Could you check a few things on this model? Use its own coordinates, in mm. Coordinates: 2 decimals unless noted, no trailing zeros. Order: outer loops, then holes, each group sorted by start corner. A loop starts at its lowest first (then second) coordinate and runs counter-clockwise, first axis right, second up. Notation, with made-up numbers: (-14.75, -37.75) - (10.25, -37.75) arc R26 cw to (10.25, -18.75) - close; hole circle Ø2 at (6, 48). An arc over 180 degrees is marked (long way). Answer as CSV lines item,"result". Start each with the question number.
1. I want a section at A-A, the plane x = 6.5. List the corners of the cut face in (y, z) for me, and give its area (3 significant figures).
2. For pin 1 (3 mm diameter, centred on x = -46.5, z = -42, fed in from -Y); pin 2 (1.5 mm diameter, centred on y = 8.5, z = -21, fed in from -X); pin 3 (6 mm diameter, centred on x = 30.5, y = 11.5, fed in from +Z); pin 4 (10 mm diameter, centred on x = -22, y = 11.5, fed in from -Z), each with a flat end and sliding along its axis, tell me the tip position at first contact or that it passes through.
3. I want a section at B-B, the plane x = -24.5. List the corners of the cut face in (y, z) for me.
4. I need wall thicknesses on probe 1 along Z at (x, y) = (-27.5, 21.25); probe 2 along X at (y, z) = (9.75, -13.5); probe 3 along X at (y, z) = (4.5, 47). Which ranges of each line are inside material? Lowest first, please.
from build123d import *

# Parameters (mm, degrees)
SKETCH1_R           = 62.5
BOSS_EXTRUDE1_DEPTH = 25
CAVITY1_DEPTH       = 25


# Read off the part's stored shape, not the designer's step: Cavity1
with BuildPart() as part:
    # Sketch1 → Boss-Extrude1 (new body)
    with BuildSketch(Plane(origin=(0, 0, 0), x_dir=(1, 0, 0), z_dir=(0, 1, 0))):
        with Locations(Location((0, 0, 0), (0, 0, 270))):
            Circle(SKETCH1_R)
    extrude(amount=BOSS_EXTRUDE1_DEPTH)

    # Cavity1 outline → Cavity1 (cut)
    with BuildSketch(Plane(origin=(0, 0, 0), x_dir=(1, 0, 0), z_dir=(0, 1, 0))):
        with BuildLine():
            Line((16.350867892, -49.873660473), (20.022970331, -51.745036944))
            ThreePointArc((20.022970331, -51.745036944), (24.456878574, -49.800038203), (28.704396647, -47.476000203))
            Line((28.704396647, -47.476000203), (29.464309883, -43.425207924))
            ThreePointArc((29.464309883, -43.425207924), (30.217762384, -42.903777412), (30.961999914, -42.369276757))
            Line((30.961999914, -42.369276757), (35.032663999, -43.014319485))
            ThreePointArc((35.032663999, -43.014319485), (38.648523661, -39.79436276), (41.969986165, -36.271516008))
            Line((41.969986165, -36.271516008), (41.440942946, -32.18415751))
            ThreePointArc((41.440942946, -32.18415751), (41.996387967, -31.455417996), (42.539030133, -30.717095621))
            Line((42.539030133, -30.717095621), (46.609790903, -30.07266333))
            ThreePointArc((46.609790903, -30.07266333), (49.053656447, -25.89294042), (51.12393549, -21.5161257))
            Line((51.12393549, -21.5161257), (49.357722251, -17.792300112))
            ThreePointArc((49.357722251, -17.792300112), (49.660788964, -16.927585698), (49.94871817, -16.05771374))
            Line((49.94871817, -16.05771374), (53.621101197, -14.186887953))
            ThreePointArc((53.621101197, -14.186887953), (54.653750036, -9.456539258), (55.270192281, -4.654189691))
            Line((55.270192281, -4.654189691), (52.43969828, -1.658411006))
            ThreePointArc((52.43969828, -1.658411006), (52.460720403, -0.742365963), (52.465752134, 0.173906448))
            Line((52.465752134, 0.173906448), (55.380278979, 3.087996269))
            ThreePointArc((55.380278979, 3.087996269), (54.900628251, 7.905931261), (54.002892036, 12.66372824))
            Line((54.002892036, 12.66372824), (50.385185747, 14.63821233))
            ThreePointArc((50.385185747, 14.63821233), (50.122105488, 15.515919131), (49.843747202, 16.388900869))
            Line((49.843747202, 16.388900869), (51.715123672, 20.061003308))
            ThreePointArc((51.715123672, 20.061003308), (49.770124931, 24.49491155), (47.446086932, 28.742429624))
            Line((47.446086932, 28.742429624), (43.395294653, 29.50234286))
            ThreePointArc((43.395294653, 29.50234286), (42.87386414, 30.255795361), (42.339363485, 31.000032891))
            Line((42.339363485, 31.000032891), (42.984406214, 35.070696976))
            ThreePointArc((42.984406214, 35.070696976), (39.764449489, 38.686556638), (36.241602736, 42.008019142))
            Line((36.241602736, 42.008019142), (32.154244239, 41.478975923))
            ThreePointArc((32.154244239, 41.478975923), (31.425504725, 42.034420944), (30.68718235, 42.57706311))
            Line((30.68718235, 42.57706311), (30.042750059, 46.64782388))
            ThreePointArc((30.042750059, 46.64782388), (25.863027148, 49.091689424), (21.486212429, 51.161968467))
            Line((21.486212429, 51.161968467), (17.762386841, 49.395755228))
            ThreePointArc((17.762386841, 49.395755228), (16.897672427, 49.698821941), (16.027800469, 49.986751147))
            Line((16.027800469, 49.986751147), (14.156974682, 53.659134174))
            ThreePointArc((14.156974682, 53.659134174), (9.426625987, 54.691783013), (4.62427642, 55.308225258))
            Line((4.62427642, 55.308225258), (1.628497735, 52.477731257))
            ThreePointArc((1.628497735, 52.477731257), (0.712452692, 52.49875338), (-0.20381972, 52.503785111))
            Line((-0.20381972, 52.503785111), (-3.11790954, 55.418311956))
            ThreePointArc((-3.11790954, 55.418311956), (-7.935844532, 54.938661228), (-12.693641511, 54.040925013))
            Line((-12.693641511, 54.040925013), (-14.668125602, 50.423218724))
            ThreePointArc((-14.668125602, 50.423218724), (-15.545832402, 50.160138465), (-16.41881414, 49.881780179))
            Line((-16.41881414, 49.881780179), (-20.090916579, 51.753156649))
            ThreePointArc((-20.090916579, 51.753156649), (-24.524824822, 49.808157908), (-28.772342895, 47.484119909))
            Line((-28.772342895, 47.484119909), (-29.532256132, 43.43332763))
            ThreePointArc((-29.532256132, 43.43332763), (-30.285708633, 42.911897117), (-31.029946162, 42.377396462))
            Line((-31.029946162, 42.377396462), (-35.100610248, 43.022439191))
            ThreePointArc((-35.100610248, 43.022439191), (-38.71646991, 39.802482465), (-42.037932414, 36.279635713))
            Line((-42.037932414, 36.279635713), (-41.508889194, 32.192277216))
            ThreePointArc((-41.508889194, 32.192277216), (-42.064334215, 31.463537702), (-42.606976382, 30.725215327))
            Line((-42.606976382, 30.725215327), (-46.677737151, 30.080783036))
            ThreePointArc((-46.677737151, 30.080783036), (-49.121602695, 25.901060125), (-51.191881738, 21.524245406))
            Line((-51.191881738, 21.524245406), (-49.425668499, 17.800419818))
            ThreePointArc((-49.425668499, 17.800419818), (-49.728735212, 16.935705404), (-50.016664419, 16.065833446))
            Line((-50.016664419, 16.065833446), (-53.689047445, 14.195007659))
            ThreePointArc((-53.689047445, 14.195007659), (-54.721696284, 9.464658964), (-55.33813853, 4.662309397))
            Line((-55.33813853, 4.662309397), (-52.507644528, 1.666530712))
            ThreePointArc((-52.507644528, 1.666530712), (-52.528666651, 0.750485669), (-52.533698382, -0.165786743))
            Line((-52.533698382, -0.165786743), (-55.448225228, -3.079876563))
            ThreePointArc((-55.448225228, -3.079876563), (-54.968574499, -7.897811555), (-54.070838284, -12.655608534))
            Line((-54.070838284, -12.655608534), (-50.453131995, -14.630092625))
            ThreePointArc((-50.453131995, -14.630092625), (-50.190051736, -15.507799425), (-49.91169345, -16.380781163))
            Line((-49.91169345, -16.380781163), (-51.783069921, -20.052883602))
            ThreePointArc((-51.783069921, -20.052883602), (-49.83807118, -24.486791845), (-47.51403318, -28.734309918))
            Line((-47.51403318, -28.734309918), (-43.463240901, -29.494223155))
            ThreePointArc((-43.463240901, -29.494223155), (-42.941810389, -30.247675656), (-42.407309734, -30.991913185))
            Line((-42.407309734, -30.991913185), (-43.052352462, -35.062577271))
            ThreePointArc((-43.052352462, -35.062577271), (-39.832395737, -38.678436932), (-36.309548985, -41.999899437))
            Line((-36.309548985, -41.999899437), (-32.222190487, -41.470856217))
            ThreePointArc((-32.222190487, -41.470856217), (-31.493450973, -42.026301238), (-30.755128598, -42.568943405))
            Line((-30.755128598, -42.568943405), (-30.110696307, -46.639704174))
            ThreePointArc((-30.110696307, -46.639704174), (-25.930973397, -49.083569718), (-21.554158677, -51.153848761))
            Line((-21.554158677, -51.153848761), (-17.830333089, -49.387635522))
            ThreePointArc((-17.830333089, -49.387635522), (-16.965618675, -49.690702235), (-16.095746717, -49.978631442))
            Line((-16.095746717, -49.978631442), (-14.22492093, -53.651014468))
            ThreePointArc((-14.22492093, -53.651014468), (-9.494572235, -54.683663307), (-4.692222668, -55.300105553))
            Line((-4.692222668, -55.300105553), (-1.696443983, -52.469611551))
            ThreePointArc((-1.696443983, -52.469611551), (-0.78039894, -52.490633674), (0.135873471, -52.495665405))
            Line((0.135873471, -52.495665405), (3.049963292, -55.410192251))
            ThreePointArc((3.049963292, -55.410192251), (7.867898284, -54.930541522), (12.625695263, -54.032805307))
            Line((12.625695263, -54.032805307), (14.600179353, -50.415099018))
            ThreePointArc((14.600179353, -50.415099018), (15.477886154, -50.152018759), (16.350867892, -49.873660473))
        make_face()
    extrude(amount=CAVITY1_DEPTH, mode=Mode.SUBTRACT)


solid = part.part
Solved:
1,outline,"(0, -62.16) - (25, -62.16) - (25, -55.12) - (0, -55.12) - close; (0, 55.11) - (25, 55.11) - (25, 62.16) - (0, 62.16) - close"
1,area,"352 mm2"
2,pin 1,"stops at y = 0"
2,pin 2,"stops at x = -59.13"
2,pin 3,"stops at z = 56.12"
2,pin 4,"stops at z = -60.14"
3,outline,"(0, -57.5) - (25, -57.5) - (25, -49.82) - (0, -49.82) - close; (0, 49.81) - (25, 49.81) - (25, 57.5) - (0, 57.5) - close"
4,probe 1,"z = -56.12 to -48.23, 48.22 to 56.12"
4,probe 2,"x = -61.02 to -53.87, 52.47 to 61.02"
4,probe 3,"x = -41.2 to -29.54, 28.79 to 41.2"
